```python
from build123d import *

# Parameters (mm, degrees)
SKETCH_1_R       = 170
SKETCH_1_R_2     = 15
SKETCH_1_R_3     = 5
EXTRUDE_1_DEPTH  = 1.5
MM_2_D           = 1
MM_2_DEPTH       = 12.4
MM_2_CSINK_D     = 12.8
MM_2_CSINK_ANGLE = 90
MM_2_TIP         = 0.30043031


with BuildPart() as part:
    # 草图1 → 凸台-拉伸1 (new, symmetric)
    with BuildSketch(Plane(origin=(0, 0, 0), x_dir=(1, 0, 0), z_dir=(0, 1, 0))):
        with Locations(Location((0, 0, 0), (0, 0, 270))):
            Circle(SKETCH_1_R)
        with Locations(Location((0, 0, 0), (0, 0, 270))):
            Circle(SKETCH_1_R_2, mode=Mode.SUBTRACT)
        with Locations(Location((-30, 0, 0), (0, 0, 270))):
            Circle(SKETCH_1_R_3, mode=Mode.SUBTRACT)
        with Locations(Location((0, 30, 0), (0, 0, 270))):
            Circle(SKETCH_1_R_3, mode=Mode.SUBTRACT)
        with Locations(Location((30, 0, 0), (0, 0, 270))):
            Circle(SKETCH_1_R_3, mode=Mode.SUBTRACT)
        with Locations(Location((0, -30, 0), (0, 0, 270))):
            Circle(SKETCH_1_R_3, mode=Mode.SUBTRACT)
    extrude(amount=EXTRUDE_1_DEPTH, both=True)

    # 大小mm 暗销孔2
    with Locations(Plane(origin=(0, 1.5, 0), x_dir=(1, 0, 0), z_dir=(0, 1, 0))):
        with Locations((-30, 0), (0, 30), (30, 0), (0, -30)):
            CounterSinkHole(MM_2_D / 2, MM_2_CSINK_D / 2, depth=MM_2_DEPTH, counter_sink_angle=MM_2_CSINK_ANGLE)
            with Locations((0, 0, -(MM_2_DEPTH + MM_2_TIP / 2))):  # 118° drill point
                Cone(0, MM_2_D / 2, MM_2_TIP, mode=Mode.SUBTRACT)


solid = part.part
```
The model under review builds one solid part; all positions refer to its coordinate system, in mm. Round coordinates to 2 decimals unless told otherwise and drop trailing zeros. Order: outer loops, then holes, each group sorted by start corner. A loop starts at its lowest first (then second) coordinate and runs counter-clockwise, first axis right, second up. Notation, with made-up numbers: M 65,43 L 103,43 A20 ccw 103,55 Z; hole C 61.5,1 d3. An arc over 180 degrees is marked long. Use a Markdown table: item, result.
1) Insertion check: pin 1 (1 mm diameter, centred on x = 76, y = 0, fed in from -Z); pin 2 (11.5 mm diameter, centred on x = 0, z = -30, fed in from +Y). Each pin has a flat end and moves straight along its axis. Give the tip position at first contact, or say it passes through.
Report:
| item | result |
|---|---|
| pin 1 | z = -152.31 |
| pin 2 | y = 0.85 |
2) Wall thickness on line 1 along X through (y, z) = (0, 0); line 2 along Z through (x, y) = (30, -0.95): over which ranges is each line inside the solid? List them lowest first. Write a range as [from, to].
Report:
| item | result |
|---|---|
| line 1 | [-170, -35], [-25, -15], [15, 25], [35, 170] |
| line 2 | [-167.33, -5], [5, 167.33] |
3) Draft analysis for pull direction X (two halves, no side actions). For faces 1 (the face through (-103.44, 0.02, -134.91)), 2 (the face through (-34.88, -0.71, -1.08)), 3 (the face through (2, 1.5, -40)), state which applies: released by +X, released by -X, zero draft, split by the parting line, or undercut.
Report:
| item | result |
|---|---|
| face 1 | split by the parting line |
| face 2 | undercut |
| face 3 | zero draft |
4) Consider section B-B (y = -0.45). Write out the cut boundary in (x, z), then the cut area to 3 significant figures.
Report:
| item | result |
|---|---|
| outline | C 0,0 d340; hole C -30,0 d10; hole C 0,0 d30; hole C 0,-30 d10; hole C 0,30 d10; hole C 30,0 d10 |
| area | 89,800 mm^2 |
5) Consider section D-D (z = 90.5). Write out the cut boundary in (x, y), then the cut area to 3 significant figures.
Report:
| item | result |
|---|---|
| outline | M -143.91,-1.5 L 143.91,-1.5 L 143.91,1.5 L -143.91,1.5 Z |
| area | 863 mm^2 |
6) Consider section A-A (z = 0). Write out the cut boundary in (x, y).
Report:
| item | result |
|---|---|
| outline | M -170,-1.5 L -35,-1.5 L -35,0.1 L -36.4,1.5 L -170,1.5 Z; M -25,-1.5 L -15,-1.5 L -15,1.5 L -23.6,1.5 L -25,0.1 Z; M 15,-1.5 L 25,-1.5 L 25,0.1 L 23.6,1.5 L 15,1.5 Z; M 35,-1.5 L 170,-1.5 L 170,1.5 L 36.4,1.5 L 35,0.1 Z |
7) Consider section C-C (x = -30). Write out the cut boundary in (y, z), then the cut area to 3 significant figures.
Report:
| item | result |
|---|---|
| outline | M -1.5,-167.33 L 1.5,-167.33 L 1.5,-6.4 L 0.1,-5 L -1.5,-5 Z; M -1.5,5 L 0.1,5 L 1.5,6.4 L 1.5,167.33 L -1.5,167.33 Z |
| area | 972 mm^2 |
